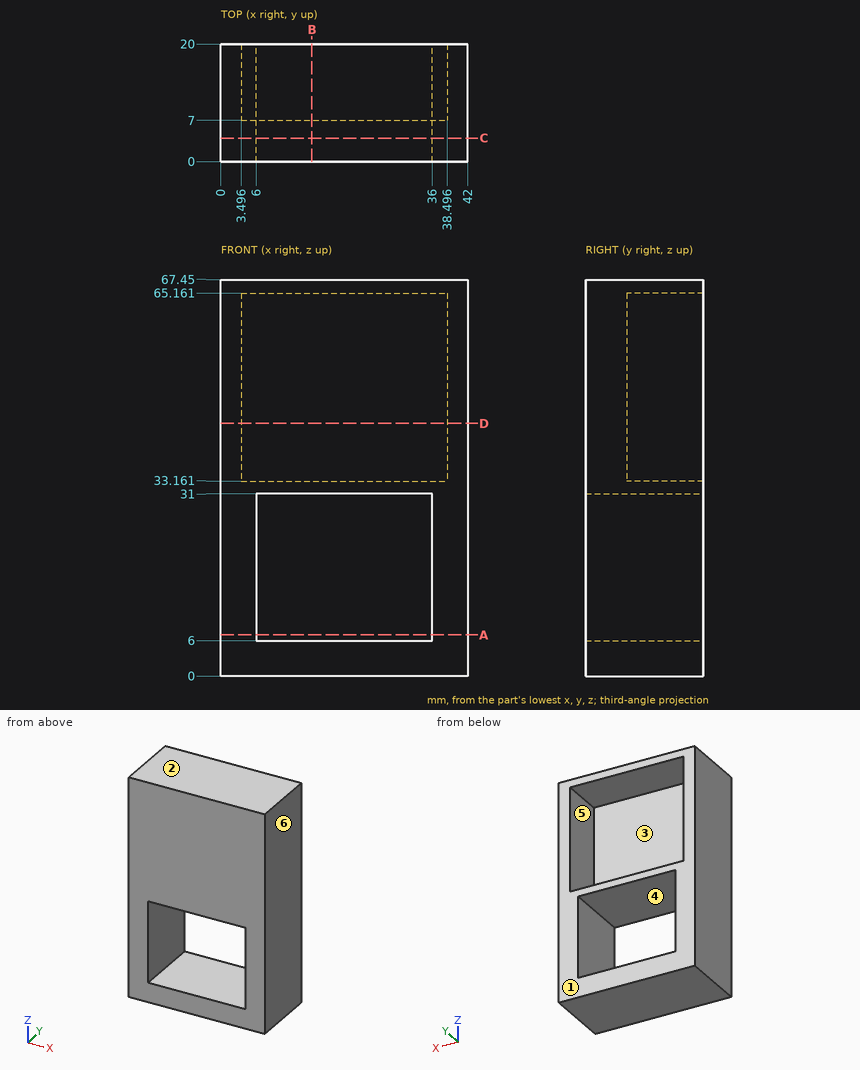
Answer from the drawing. Dimensions are ordinates in mm from the lowest x, y and z of the part. A direction names the side the tool comes from. Round coordinates to 2 decimals unless told otherwise and drop trailing zeros. Loops run counter-clockwise (first coordinate to the right, second up) from the corner with the lowest first, then second, coordinate; pieces in that order, holes last. Notation, with made-up numbers: (85, 60) - (99, 60) arc R33 ccw to (99, 96) - close; hole circle Ø10 at (77, 79.25). An arc over 180 degrees is marked (long way). Return JSON: item names as keys, results as strings. Group by question number.
1. The part is cut by section B-B on x = 15.5. Determine the outline of the cut face in (y, z).
2. Consider probe 1 along Z at (x, y) = (35, 11); probe 2 along X at (y, z) = (10.5, 20); probe 3 along X at (y, z) = (10.25, 43). Determine where each line is inside the solid, lowest interval first.
3. This flat-tipped pin is pushed along its axis until it touches: P1, Ø9.5, axis at x = 26, z = 55.5, coming from the +Y side. Where does it stop, or does it pass through?
4. The mould has two halves that part along Z. Classify the marked faces 1, 2 and 3: pulls with the +Z half, pulls with the -Z half, needs draft (parallel to the pull), parting line crosses it, or undercut.
5. Which of the six approach directions +Z, -Z, +X, -X, +Y, -Y give full straight-line access (tool end or side, diameter ignored) to the marked faces 4, 5 and 6?
6. The part is cut by section A-A on z = 7. Determine the outline of the cut face in (x, y), then the cut area to 3 significant figures.
7. The part is cut by section D-D on z = 43. Determine the outline of the cut face in (x, y), then the cut area to 3 significant figures.
8. The part is cut by section C-C on y = 4. Determine the outline of the cut face in (x, z).
Resolved:
{
 "1": {"outline": "(0, 0) - (20, 0) - (20, 6) - (0, 6) - close; (0, 31) - (20, 31) - (20, 33.16) - (7, 33.16) - (7, 65.16) - (20, 65.16) - (20, 67.45) - (0, 67.45) - close"},
 "2": {"probe 1": "z = 0 to 6, 31 to 33.16, 65.16 to 67.45", "probe 2": "x = 0 to 6, 36 to 42", "probe 3": "x = 0 to 3.5, 38.5 to 42"},
 "3": {"P1": "stops at y = 7"},
 "4": {"face 1": "needs draft", "face 2": "pulls with the +Z half", "face 3": "undercut"},
 "5": {"face 4": "+Y, -Y", "face 5": "+Y", "face 6": "+Z, -Z, +X, +Y, -Y"},
 "6": {"outline": "(0, 0) - (6, 0) - (6, 20) - (0, 20) - close; (36, 0) - (42, 0) - (42, 20) - (36, 20) - close", "area": "240 mm²"},
 "7": {"outline": "(0, 0) - (42, 0) - (42, 20) - (38.5, 20) - (38.5, 7) - (3.5, 7) - (3.5, 20) - (0, 20) - close", "area": "385 mm²"},
 "8": {"outline": "(0, 0) - (42, 0) - (42, 67.45) - (0, 67.45) - close; hole (6, 6) - (36, 6) - (36, 31) - (6, 31) - close"}
}
